```python
from build123d import *

# Parameters (mm, degrees)
F0_R     = 10
F1_DEPTH = 2
F3_DEPTH = 2.001
F6_W     = 6.3617299311
F6_H     = 2
F7_DEPTH = 1


with BuildPart() as f1:
    # F0 (on Top) → F1 (new body)
    with BuildSketch(Plane.XY):
        Circle(F0_R)
    extrude(amount=F1_DEPTH)

    # F2 (on face) → F3 (cut, through all)
    with BuildSketch(Plane.XY.offset(2)):
        with BuildLine():
            ThreePointArc((-4.7696960071, 1.5), (-3.5355339059, 3.5355339059), (-1.5, 4.7696960071))
            Line((-1.5, 4.7696960071), (-1.5, 9.8868599666))
            ThreePointArc((-1.5, 9.8868599666), (-7.0710678119, 7.0710678119), (-9.8868599666, 1.5))
            Line((-9.8868599666, 1.5), (-4.7696960071, 1.5))
        make_face()
        with BuildLine():
            ThreePointArc((1.5, 4.7696960071), (3.5355339059, 3.5355339059), (4.7696960071, 1.5))
            Line((4.7696960071, 1.5), (9.8868599666, 1.5))
            ThreePointArc((9.8868599666, 1.5), (7.0710678119, 7.0710678119), (1.5, 9.8868599666))
            Line((1.5, 9.8868599666), (1.5, 4.7696960071))
        make_face()
        with BuildLine():
            Line((9.8868599666, -1.5), (4.7696960071, -1.5))
            ThreePointArc((4.7696960071, -1.5), (3.5355339059, -3.5355339059), (1.5, -4.7696960071))
            Line((1.5, -4.7696960071), (1.5, -9.8868599666))
            ThreePointArc((1.5, -9.8868599666), (7.0710678119, -7.0710678119), (9.8868599666, -1.5))
        make_face()
        with BuildLine():
            Line((-1.5, -9.8868599666), (-1.5, -4.7696960071))
            ThreePointArc((-1.5, -4.7696960071), (-3.5355339059, -3.5355339059), (-4.7696960071, -1.5))
            Line((-4.7696960071, -1.5), (-9.8868599666, -1.5))
            ThreePointArc((-9.8868599666, -1.5), (-7.0710678119, -7.0710678119), (-1.5, -9.8868599666))
        make_face()
    extrude(amount=-F3_DEPTH, mode=Mode.SUBTRACT)

    # F4 (on Right) → F5 (revolve)
    with BuildSketch(Plane.YZ):
        with BuildLine():
            Line((4.5, 0), (0, 0))
            Line((0, 0), (0, -5))
            ThreePointArc((0, -5), (3.2165335145, -3.369880163), (4.5, 0))
        make_face()
    revolve(axis=Axis((0, 0, 2.0248414949), (0, 0, 1)))

    # F6 (on Front) → F7 (cut, symmetric)
    with BuildSketch(Plane.XZ):
        with Locations((0, -5.0499816425)):
            Rectangle(F6_W, F6_H)
    extrude(amount=F7_DEPTH, both=True, mode=Mode.SUBTRACT)


solid = f1.part
```
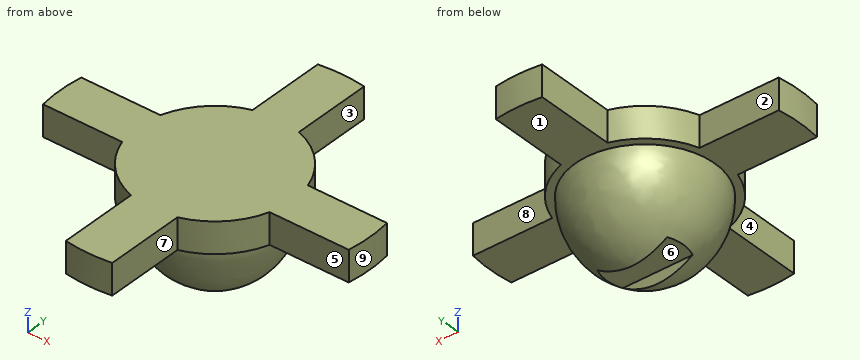
Input: part model. Units: mm. Frame: model coordinates. Face numbers are marked on the shaded views. A direction names the side the tool comes from. Give positions to 0.01 mm unless a question says otherwise; leave off trailing zeros. Order: outer loops, then holes, each group sorted by start corner. A loop starts at its lowest first (then second) coordinate and runs counter-clockwise, first axis right, second up. Notation, with made-up numbers: (14, 71.5) - (40, 71.5) arc R11 cw to (40, 80.5) - close; hole circle Ø5 at (6, 50.25). An arc over 180 degrees is marked (long way). Use a Markdown table: item, result.
(1) Line query: line 1 (Y direction, x = -0.25, z = -4.5); line 2 (Z direction, x = -0.5, y = 5.25); line 3 (X direction, y = 8, z = 1). Output: solid intervals per line, ascending. Write a range as from..to.
Computed values:
| item | result |
|---|---|
| line 1 | y = -1.71..-1, 1..1.71 |
| line 2 | z = 0..2 |
| line 3 | x = -1.5..1.5 |
(2) Section query A-A (z = 0.75). Output: boundary loops of the cut face in (x, y).
Computed values:
| item | result |
|---|---|
| outline | (-9.89, -1.5) - (-4.77, -1.5) arc R5 ccw to (-1.5, -4.77) - (-1.5, -9.89) arc R10 ccw to (1.5, -9.89) - (1.5, -4.77) arc R5 ccw to (4.77, -1.5) - (9.89, -1.5) arc R10 ccw to (9.89, 1.5) - (4.77, 1.5) arc R5 ccw to (1.5, 4.77) - (1.5, 9.89) arc R10 ccw to (-1.5, 9.89) - (-1.5, 4.77) arc R5 ccw to (-4.77, 1.5) - (-9.89, 1.5) arc R10 ccw to start |
(3) Access query for the marked faces 1, 2, 3, 4 and 5. Directions: +Z, -Z, +X, -X, +Y, -Y. A direction counts if a zero-diameter tool reaches every point of the face in a straight line with its end or side. Return the directions, or none.
Computed values:
| item | result |
|---|---|
| face 1 | -Z |
| face 2 | +Z, -Z, -X, +Y |
| face 3 | +Z, -Z, +X, +Y |
| face 4 | +Z, -Z, -X, -Y |
| face 5 | +Z, -Z, +X, -Y |
(4) Draft query along Y for the marked faces 6, 7, 8 and 9. Return one class per face: released by +Y, released by -Y, zero draft, split by the parting line, or undercut.
Computed values:
| item | result |
|---|---|
| face 6 | undercut |
| face 7 | zero draft |
| face 8 | released by +Y |
| face 9 | split by the parting line |
(5) Pin query (flat end, axial travel): pin 1 (0.6 mm diameter, centred on x = 7.5, z = 1, fed in from +Y); pin 2 (1 mm diameter, centred on y = 8, z = 1, fed in from +X); pin 3 (1 mm diameter, centred on x = 6, z = 0.5, fed in from -Y). Return the tip coordinate at first contact, or that it passes through.
Computed values:
| item | result |
|---|---|
| pin 1 | stops at y = 1.5 |
| pin 2 | stops at x = 1.5 |
| pin 3 | stops at y = -1.5 |
(6) Section query B-B (y = -8.5). Output: boundary loops of the cut face in (x, z), then the cut area to 3 significant figures.
Computed values:
| item | result |
|---|---|
| outline | (-1.5, 0) - (1.5, 0) - (1.5, 2) - (-1.5, 2) - close |
| area | 6.00 mm2 |
